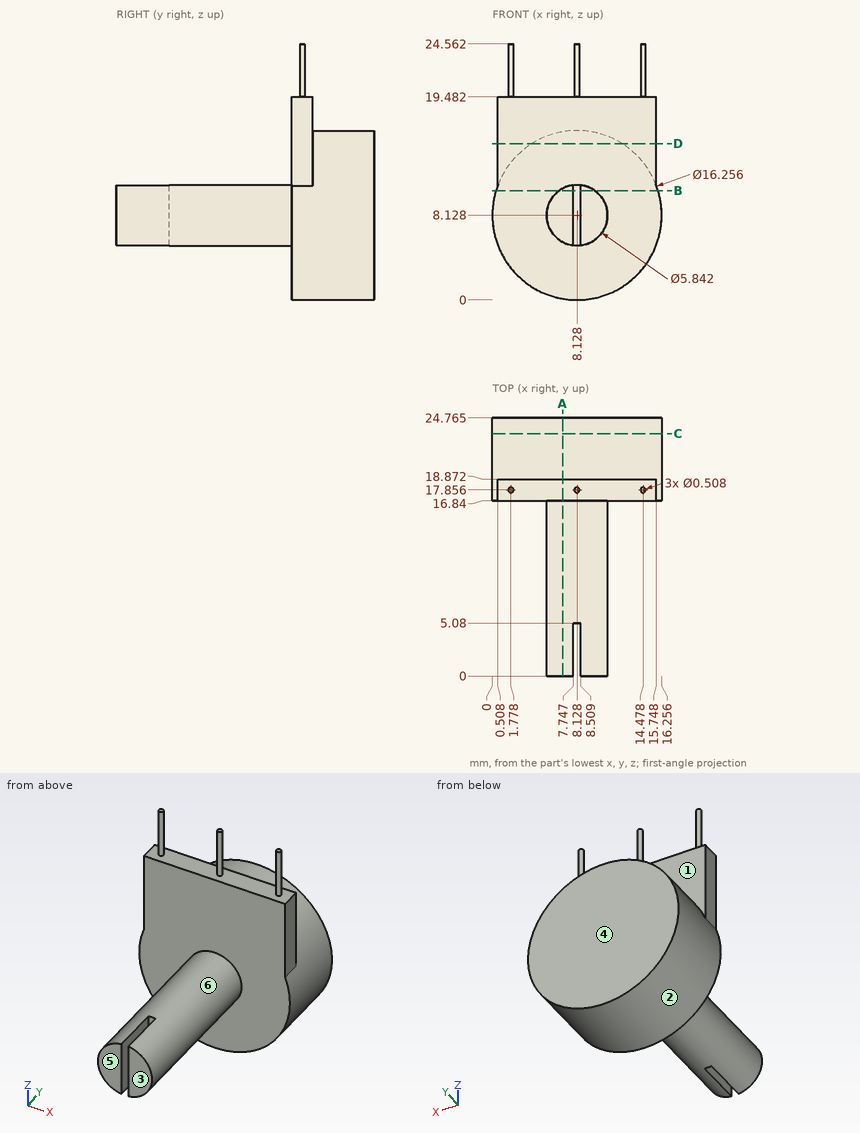
Can you work these out from the drawing? Everything is in mm from the part's minimum corner. A direction names the side the tool comes from. Give positions to 0.01 mm unless a question says otherwise; leave off trailing zeros. Order: outer loops, then holes, each group sorted by start corner. A loop starts at its lowest first (then second) coordinate and runs counter-clockwise, first axis right, second up. Notation, with made-up numbers: M 64.5,59.5 L 104.5,59.5 A17 ccw 104.5,71.5 Z; hole C -25,37 d10. An arc over 180 degrees is marked long. One line per item, written item: value.
Item 1: If we section it at C-C on y = 23.25: Write out the boundary of the cut face in (x, z), and give its area (3 significant figures).
Verdict:
outline: C 8.13,8.13 d16.26
area: 208 mm2
Item 2: If we section it at D-D on z = 15: Write out the boundary of the cut face in (x, y) (1 decimal).
Verdict:
outline: M 0.5,16.8 L 15.7,16.8 L 15.7,18.9 L 12.5,18.9 L 12.5,24.8 L 3.8,24.8 L 3.8,18.9 L 0.5,18.9 Z
Item 3: If we section it at A-A on x = 6.75: Write out the boundary of the cut face in (y, z) (1 decimal), and give its area (4 significant figures).
Verdict:
outline: M 0,5.6 L 16.8,5.6 L 16.8,0.1 L 24.8,0.1 L 24.8,16.1 L 18.9,16.1 L 18.9,19.5 L 16.8,19.5 L 16.8,10.7 L 0,10.7 Z
area: 220.5 mm2
Item 4: For pin 1 (2 mm diameter, centred on y = 17.5, z = 14.5, fed in from +X); pin 2 (3 mm diameter, centred on x = 12, y = 20.5, fed in from -Z); pin 3 (1 mm diameter, centred on y = 21.5, z = 3.5, fed in from +X), each with a flat end and sliding along its axis, tell me the tip position at first contact or that it passes through.
Verdict:
pin 1: x = 15.75
pin 2: z = 0.35
pin 3: x = 15.13
Item 5: For the marked faces 1, 2 and 3, which set-ups out of +Z, -Z, +X, -X, +Y, -Y let a thin tool reach every point of the face, with its end or its side?
Verdict:
face 1: +Z, +Y
face 2: +Y
face 3: +Z, -Z, +X, -X, -Y
Item 6: If we mould it in two halves opening along Y, with no side actions, what happens to the marked faces 4, 5 and 6? For each: pulls with the +Y half, pulls with the -Y half, needs draft (parallel to the pull), parting line crosses it, or undercut.
Verdict:
face 4: pulls with the +Y half
face 5: pulls with the -Y half
face 6: needs draft
Item 7: If we section it at B-B on z = 10.5: Write out the boundary of the cut face in (x, y) (1 decimal), and give its area (3 significant figures).
Verdict:
outline: M 0.4,16.8 L 6.4,16.8 L 6.4,0 L 7.7,0 L 7.7,5.1 L 8.5,5.1 L 8.5,0 L 9.8,0 L 9.8,16.8 L 15.9,16.8 L 15.9,24.8 L 0.4,24.8 Z
area: 177 mm2
Item 8: Please list where these lines run through material, in increasing order: line 1 (Y direction, x = 8.75, z = 2) (1 decimal); line 2 (Y direction, x = 7.75, z = 18.5); line 3 (Z direction, x = 13.5, y = 17.75).
Verdict:
line 1: 16.8 to 24.8
line 2: 16.84 to 18.87
line 3: 2.03 to 19.48
